The model under review builds one solid part; all positions refer to its coordinate system, in mm. A direction names the side the tool comes from. Round coordinates to 2 decimals unless told otherwise and drop trailing zeros. Order: outer loops, then holes, each group sorted by start corner. A loop starts at its lowest first (then second) coordinate and runs counter-clockwise, first axis right, second up. Notation, with made-up numbers: (58.25, 17.5) -> (97.25, 17.5) arc R13 ccw to (97.25, 29.5) -> close; hole circle Ø7 at (5, 30). An arc over 180 degrees is marked (long way). Put each result on its own line as item: value. Start each with the question number.
from build123d import *

# Parameters (mm, degrees)
SKETCH1_W           = 92
SKETCH1_H           = 31
BOSS_EXTRUDE1_DEPTH = 46
SKETCH2_R           = 103
SKETCH2_R_2         = 73
CUT_EXTRUDE1_DEPTH  = 47
SKETCH7_R           = 1.2
CUT_EXTRUDE5_DEPTH  = 47
CUT_EXTRUDE2_DEPTH  = 47
SKETCH5_R           = 42.5
CUT_EXTRUDE4_DEPTH  = 17.103780853
CUT_EXTRUDE6_START  = -2
CUT_EXTRUDE6_DEPTH  = 2.2


with BuildPart() as part:
    # Sketch1 → Boss-Extrude1 (new body)
    with BuildSketch(Plane(origin=(0, 0, 0), x_dir=(1, 0, 0), z_dir=(0, 1, 0))):
        Rectangle(SKETCH1_W, SKETCH1_H)
    extrude(amount=BOSS_EXTRUDE1_DEPTH)

    # Sketch2 → Cut-Extrude1 (cut, through all)
    with BuildSketch(Plane(origin=(0, 46, 0), x_dir=(1, 0, 0), z_dir=(0, 1, 0))):
        with Locations((0, -53.5)):
            Circle(SKETCH2_R)
        with Locations((0, -53.5)):
            Circle(SKETCH2_R_2, mode=Mode.SUBTRACT)
    extrude(amount=-CUT_EXTRUDE1_DEPTH, mode=Mode.SUBTRACT)

    # Sketch7 → Cut-Extrude5 (cut, through all)
    with BuildSketch(Plane.XZ):
        with Locations((-32, -7.5)):
            Circle(SKETCH7_R)
        with Locations((32, -7.5)):
            Circle(SKETCH7_R)
    extrude(amount=-CUT_EXTRUDE5_DEPTH, mode=Mode.SUBTRACT)

    # Sketch3 → Cut-Extrude2 (cut, through all)
    with BuildSketch(Plane(origin=(0, 46, 0), x_dir=(1, 0, 0), z_dir=(0, 1, 0))):
        with BuildLine():
            Line((-37.855118544, 5.5), (37.855118544, 5.5))
            ThreePointArc((37.855118544, 5.5), (0, -123.6), (-37.855118544, 5.5))
        make_face()
    extrude(amount=-CUT_EXTRUDE2_DEPTH, mode=Mode.SUBTRACT)

    # Sketch5 → Cut-Extrude4 (cut, through all)
    with BuildSketch(Plane(origin=(0, 0, -15.5), x_dir=(-1, 0, 0), z_dir=(0, 0, -1))):
        with Locations((0, 46)):
            Circle(SKETCH5_R)
    extrude(amount=-CUT_EXTRUDE4_DEPTH, mode=Mode.SUBTRACT)

    # Sketch8 → Cut-Extrude6 (cut)
    with BuildSketch(Plane.XZ.offset(CUT_EXTRUDE6_START)):
        Polygon((-34.523561667, -7.229062977), (-33.183568052, -9.55), (-30.816431948, -9.55), (-29.904759513, -7.970937023), (-29.904759513, -4.97225781), (-34.523561667, -4.97225781), align=None)
        Polygon((29.904759513, -4.97225781), (29.904759513, -7.970937023), (30.816431948, -9.55), (33.183568052, -9.55), (34.523561667, -7.229062977), (34.523561667, -4.97225781), align=None)
    extrude(amount=-CUT_EXTRUDE6_DEPTH, mode=Mode.SUBTRACT)


solid = part.part
Q1. Clearance check with flat-ended pins moving along their axes: pin 1 Ø1.5 at (x, z) = (29.5, -9.5) entering from +Y; pin 2 Ø8 at (x, z) = (16, -5.5) entering from +Y; pin 3 Ø3 at (x, z) = (33.5, -8) entering from +Y; pin 4 Ø1.9 at (x, z) = (-32, -7.5) entering from +Y. State where each tip first meets the part, or that it passes through.
Q2. Draft analysis for pull direction Z (two halves, no side actions). For faces 4 (the face through (-30.855, 0.986, -7.14)), 5 (the face through (-30.367, 3.085, -8.772)), 6 (the face through (-29.905, 3, -7)), state which applies: +Z half, -Z half, draft (parallel to the pull), parting line (faces both ways), or undercut.
Q3. For faces 1 (the face through (41.98, 18.21, -2.64)), 2 (the face through (0, 3, -15.5)), 3 (the face through (34.524, 3, -6)), list the 3-axis set-ups (+Z, -Z, +X, -X, +Y, -Y) from which the entire face can be reached by the end or side of a thin tool; tool diameter is ignored.
Q4. Take a section at B-B on x = -32. Give the boundary of the cut face in (y, z), and give its area (3 significant figures).
Q5. Take a section at D-D on x = 10.5. Give the boundary of the cut face in (y, z).
Q6. Wall thickness on probe 1 along X at (y, z) = (8.25, -7.5); probe 2 along X at (y, z) = (11.75, -7.5); probe 3 along X at (y, z) = (31.5, -7.25): over which ranges is each line inside the solid? List them lowest first. Write a range as [from, to].
Q7. Take a section at A-A on y = 36. Give the boundary of the cut face in (x, z).
Q8. Take a section at C-C on z = -12.5. Give the boundary of the cut face in (x, y).
Calculated:
1. pin 1: stops at y = 16.15
1. pin 2: stops at y = 8.5
1. pin 3: stops at y = 21.89
1. pin 4: passes through
2. face 4: undercut
2. face 5: +Z half
2. face 6: draft
3. face 1: +Z, +Y, -Y
3. face 2: -Z, +X, -X, +Y, -Y
3. face 3: +Z
4. outline: (0, -12.11) -> (18.03, -12.11) -> (18.03, -8.7) -> (4.2, -8.7) -> (4.2, -9.55) -> (2, -9.55) -> (2, -8.7) -> (0, -8.7) -> close; (0, -6.3) -> (2, -6.3) -> (2, -5.5) -> (0, -5.5) -> close; (4.2, -6.3) -> (18.03, -6.3) -> (18.03, -5.5) -> (4.2, -5.5) -> close
4. area: 72.3 mm²
5. outline: (0, -15.5) -> (4.82, -15.5) -> (4.82, -5.5) -> (0, -5.5) -> close
6. probe 1: x = [-40.1, -33.2], [-30.8, -19.52], [19.52, 30.8], [33.2, 40.1]
6. probe 2: x = [-40.1, -33.2], [-30.8, -25.16], [25.16, 30.8], [33.2, 40.1]
6. probe 3: x = [-40.48, -39.95], [39.95, 40.48]
7. outline: (-46, -3.18) arc R73 ccw to (-41.31, -6.69) -> (-41.31, -3.14) arc R70.1 cw to (-46, 0.6) -> close; (41.31, -6.69) arc R73 ccw to (46, -3.18) -> (46, 0.6) arc R70.1 cw to (41.31, -3.14) -> close
8. outline: (-31.19, 0) -> (31.19, 0) -> (31.19, 17.13) arc R42.5 cw to (-31.19, 17.13) -> close
